Here's how the part is built. I have some questions about the finished solid (model axes, mm). A direction names the side the tool comes from. Coordinates: 2 decimals unless noted, no trailing zeros. Loops run counter-clockwise (first coordinate to the right, second up) from the corner with the lowest first, then second, coordinate; pieces in that order, holes last. Notation, with made-up numbers: (15, 12.5) - (68, 12.5) arc R32 ccw to (68, 50.5) - close; hole circle Ø4 at (1, -10.5). An arc over 180 degrees is marked (long way). Use a Markdown table: item, result.
```python
from build123d import *

# Parameters (mm, degrees)
SKETCH1_R               = 30
BOSS_EXTRUDE1_DEPTH     = 10
SKETCH2_R               = 10
BOSS_EXTRUDE2_DEPTH     = 65.1
SKETCH2_2_R             = 10
BOSS_EXTRUDE3_DEPTH     = 20
SKETCH5_R               = 5
CUT_EXTRUDE1_DEPTH      = 87.255492579
SKETCH6_R               = 2
CUT_EXTRUDE2_DEPTH      = 78.704633067
CIRPATTERN1_COUNT       = 2
CIRPATTERN1_ANGLE       = 90
CUT_EXTRUDE3_DEPTH      = 87.255492666
CUT_EXTRUDE3_DEPTH_BACK = 87.255492666
SKETCH7_R               = 2
SKETCH9_W               = 11
SKETCH9_H               = 3
CUT_EXTRUDE5_DEPTH      = 10
SKETCH10_R              = 3.5
CUT_EXTRUDE6_DEPTH      = 8
SKETCH17_R              = 7.355644599
BOSS_EXTRUDE4_DEPTH     = 25
SKETCH18_R              = 3
CUT_EXTRUDE7_DEPTH      = 15
BOSS_EXTRUDE5_START     = 10
BOSS_EXTRUDE5_DEPTH     = 10


with BuildPart() as part:
    # Sketch1 → Boss-Extrude1 (new body)
    with BuildSketch(Plane.XY):
        Circle(SKETCH1_R)
    extrude(amount=BOSS_EXTRUDE1_DEPTH)

    # Sketch2 → Boss-Extrude2 (add)
    with BuildSketch(Plane(origin=(0, 0, 0), x_dir=(-1, 0, 0), z_dir=(0, 0, -1))):
        Circle(SKETCH2_R)
    extrude(amount=BOSS_EXTRUDE2_DEPTH)

    # Sketch2_2 → Boss-Extrude3 (add)
    with BuildSketch(Plane(origin=(0, 0, 0), x_dir=(-1, 0, 0), z_dir=(0, 0, -1))):
        Circle(SKETCH2_2_R)
    extrude(amount=BOSS_EXTRUDE3_DEPTH)

    # Sketch5 → Cut-Extrude1 (cut, through all)
    with BuildSketch(Plane(origin=(0, 0, -65.1), x_dir=(-1, 0, 0), z_dir=(0, 0, -1))):
        Circle(SKETCH5_R)
    extrude(amount=-CUT_EXTRUDE1_DEPTH, mode=Mode.SUBTRACT)

    # Sketch6 → Cut-Extrude2 (cut, symmetric)
    with BuildSketch(Plane(origin=(0, 0, 0), x_dir=(1, 0, 0), z_dir=(0, 1, 0))):
        with Locations(Location((0, 17.6, 0), (0, 0, 270))):
            Circle(SKETCH6_R)
    cut_extrude2 = extrude(amount=CUT_EXTRUDE2_DEPTH, both=True, mode=Mode.SUBTRACT)

    # CirPattern1: Cut-Extrude2 ×2 about axis
    cirpattern1_axis = Axis((0, 0, -65.1), (0, 0, 1))
    for i in range(1, CIRPATTERN1_COUNT):
        add(cut_extrude2.rotate(cirpattern1_axis, i * CIRPATTERN1_ANGLE / (CIRPATTERN1_COUNT - 1)), mode=Mode.SUBTRACT)

    # Sketch7 → Cut-Extrude3 (cut, two sides: drawn at the far end of the back side and taken through both)
    with BuildSketch(Plane.XY.offset(10).offset(-CUT_EXTRUDE3_DEPTH_BACK)):
        with Locations((0, 16)):
            Circle(SKETCH7_R)
        with Locations((11.313708499, 11.313708499)):
            Circle(SKETCH7_R)
        with Locations((16, 0)):
            Circle(SKETCH7_R)
        with Locations((11.313708499, -11.313708499)):
            Circle(SKETCH7_R)
        with Locations((0, -16)):
            Circle(SKETCH7_R)
        with Locations((-11.313708499, -11.313708499)):
            Circle(SKETCH7_R)
        with Locations((-16, 0)):
            Circle(SKETCH7_R)
        with Locations((-11.313708499, 11.313708499)):
            Circle(SKETCH7_R)
    extrude(amount=CUT_EXTRUDE3_DEPTH + CUT_EXTRUDE3_DEPTH_BACK, mode=Mode.SUBTRACT)

    # Sketch9 → Cut-Extrude5 (cut)
    with BuildSketch(Plane(origin=(0, 0, 0), x_dir=(-1, 0, 0), z_dir=(0, 0, -1))):
        with Locations((0, 25.5)):
            Rectangle(SKETCH9_W, SKETCH9_H)
    cut_extrude5 = extrude(amount=-CUT_EXTRUDE5_DEPTH, mode=Mode.SUBTRACT)

    # Mirror1: Cut-Extrude5 across plane
    add(cut_extrude5.mirror(Plane.ZX), mode=Mode.SUBTRACT)

    # Sketch10 → Cut-Extrude6 (cut)
    with BuildSketch(Plane(origin=(0, -30, 0), x_dir=(-1, 0, 0), z_dir=(0, -1, 0))):
        with Locations(Location((0, -4.5, 0), (0, 0, 90))):
            Circle(SKETCH10_R)
    cut_extrude6 = extrude(amount=-CUT_EXTRUDE6_DEPTH, mode=Mode.SUBTRACT)

    # Mirror2: Cut-Extrude6 across plane
    add(cut_extrude6.mirror(Plane.ZX), mode=Mode.SUBTRACT)

    # Sketch17 → Boss-Extrude4 (add)
    with BuildSketch(Plane(origin=(0, 0, -40.1), x_dir=(-1, 0, 0), z_dir=(0, 0, -1))):
        Circle(SKETCH17_R)
    extrude(amount=BOSS_EXTRUDE4_DEPTH)

    # Sketch18 → Cut-Extrude7 (cut)
    with BuildSketch(Plane(origin=(0, 0, -65.1), x_dir=(-1, 0, 0), z_dir=(0, 0, -1))):
        Circle(SKETCH18_R)
    extrude(amount=-CUT_EXTRUDE7_DEPTH, mode=Mode.SUBTRACT)

    # Sketch19 → Boss-Extrude5 (add)
    with BuildSketch(Plane(origin=(0, 0, -50.1), x_dir=(-1, 0, 0), z_dir=(0, 0, -1)).offset(BOSS_EXTRUDE5_START)):
        with BuildLine():
            Line((1.658312395, 2.5), (-1.658312395, 2.5))
            ThreePointArc((-1.658312395, 2.5), (0, 3), (1.658312395, 2.5))
        make_face()
    extrude(amount=-BOSS_EXTRUDE5_DEPTH)


solid = part.part
```
Q1. Please list where these lines run through material, in increasing order: L1, parallel to Y at x = 0, z = 4; L2, parallel to Y at x = 0, z = -11; L3, parallel to Z at x = 4.5, y = -20. Write a range as from..to.
Check values:
| item | result |
|---|---|
| L1 | -22..-18, -14..-5, 5..14, 18..22 |
| L2 | -10..-5, 5..10 |
| L3 | 0..10 |
Q2. I want a section at A-A, the plane y = 0. Give the number of separate pieces and of enclosed holes in the cut face, then the cut area to 3 significant figures.
Check values:
| item | result |
|---|---|
| separate pieces | 5 |
| enclosed holes | 0 |
| area | 1,190 mm^2 |
Q3. I want a section at B-B, the plane x = 16. Write out the boundary of the cut face in (y, z), then the cut area to 3 significant figures.
Check values:
| item | result |
|---|---|
| outline | (-25.38, 0) - (-2, 0) - (-2, 10) - (-25.38, 10) - close; (2, 0) - (25.38, 0) - (25.38, 10) - (2, 10) - close |
| area | 468 mm^2 |
Q4. If we mould it in two halves opening along X, with no side actions, what happens to faces 6 (the face through (-5.5, 25, 5)), 7 (the face through (-1.341, 23.014, 1.267)), 8 (the face through (-29.97, 1.32, 4.93)), 9 (the face through (6, 0, 10))? For each: pulls with the +X half, pulls with the -X half, needs draft (parallel to the pull), parting line crosses it, or undercut.
Check values:
| item | result |
|---|---|
| face 6 | undercut |
| face 7 | undercut |
| face 8 | parting line crosses it |
| face 9 | needs draft |
Q5. Will these pins go through, and if not, where does the flat tip stop? P1, Ø12, axis at x = -16.5, z = -48, coming from the -Y side; P2, Ø6.5, axis at x = 0, z = -17.6, coming from the -Y side; P3, Ø3.5, axis at y = 25, z = 7.5, coming from the +X side; P4, Ø1, axis at x = -7.5, z = -14.5, coming from the +Y side.
Check values:
| item | result |
|---|---|
| P1 | through |
| P2 | y = -10 |
| P3 | x = 18.96 |
| P4 | y = 7.14 |
Q6. Which directions (+Z, -Z, +X, -X, +Y, -Y) give clear straight access to the entire face, cutting with the end or side of a thin tool? Please do faces 1 (the face through (-5.5, -25, 5)), 2 (the face through (0.088, 7.332, -19.598)), 3 (the face through (-1.341, -23.014, 1.267)), 4 (the face through (0, 0, -50.1)), 5 (the face through (1.08, -4.88, -15.4)).
Check values:
| item | result |
|---|---|
| face 1 | +Z, -Z |
| face 2 | +Y, -Y |
| face 3 | -Y |
| face 4 | -Z |
| face 5 | +Z |
